For this review, take the finished solid that the model builds, in its own axes (mm). A direction names the side the tool comes from. Coordinates: 2 decimals unless noted, no trailing zeros. Loops run counter-clockwise (first coordinate to the right, second up) from the corner with the lowest first, then second, coordinate; pieces in that order, holes last. Notation, with made-up numbers: (-36.5, 67.25) -> (-24.5, 67.25) arc R17 ccw to (-24.5, 96.25) -> close; hole circle Ø5 at (8.25, -5.75). An arc over 180 degrees is marked (long way). One line per item, written item: value.
Autodesk Inventor part; units mm, degrees
ref_plane "YZ Plane" through (0, 0, 0) normal (1, 0, 0) x (0, 1, 0)
ref_plane "XZ Plane" through (0, 0, 0) normal (0, 1, 0) x (-1, 0, 0)
ref_plane "XY Plane" through (0, 0, 0) normal (0, 0, 1) x (1, 0, 0)
sketch "Sketch1" plane through (0, 0, 0) normal (0, 0, 1) x (1, 0, 0)
  line L0 (-15, 13.1624) -> (0, 13.1624) construction
  line L1 (-15, -13.1624) -> (-15, 13.1624) construction
  line L2 (0, -13.1624) -> (-15, -13.1624) construction
  line L3 (0, 13.1624) -> (0, -13.1624) construction
  circle A0 centre (20, -58.85) radius 1.2295 construction
  circle A1 centre (20, -38.35) radius 1.2295 construction
  circle A2 centre (42.1, -48.6) radius 1.2295 construction
  circle A3 centre (20, -48.6) radius 6 construction
  circle A4 centre (20, 0) radius 4 construction
  line L4 (40, 13.1624) -> (55, 13.1624) construction
  line L5 (40, -13.1624) -> (40, 13.1624) construction
  line L6 (55, -13.1624) -> (40, -13.1624) construction
  line L7 (55, 13.1624) -> (55, -13.1624) construction
  arc A5 (0, 0) -> (-15, 0) centre (-7.5, 0) ccw
  arc A6 (55, 0) -> (40, 0) centre (47.5, 0) ccw
  arc A7 (0, 0) -> (40, 0) centre (20, 0) ccw
  line L8 (53.51, -48.6) -> (3.95, -48.6) construction
  line L9 (20, -64.85) -> (43, -64.85)
  line L10 (55, 0) -> (55, -52.85)
  arc A8 (43, -64.85) -> (55, -52.85) centre (43, -52.85) ccw
  line L11 (4.8831, -54.5617) -> (-13.4793, -8.001)
  arc A9 (4.8831, -54.5617) -> (20, -64.85) centre (20, -48.6) ccw
  arc A10 (-15, 0) -> (-13.4793, -8.001) centre (6.8084, 0) ccw
  circle A11 centre (42.1, -48.6) radius 1.5
  arc A12 (19.1333, -36.7114) -> (18.1846, -38.7583) centre (42.1, -48.6) ccw
  arc A13 (21.7975, -38.0905) -> (20.9588, -39.9) centre (42.1, -48.6) ccw
  arc A14 (20.9609, -57.3051) -> (21.8001, -59.1144) centre (42.1, -48.6) ccw construction
  arc A15 (18.1869, -58.4474) -> (19.1362, -60.4941) centre (42.1, -48.6) ccw
  arc A16 (19.1362, -60.4941) -> (21.8001, -59.1144) centre (20.4681, -59.8042) ccw
  arc A17 (20.9609, -57.3051) -> (18.1869, -58.4474) centre (19.5739, -57.8763) ccw
  arc A18 (18.1846, -38.7583) -> (20.9588, -39.9) centre (19.5717, -39.3292) ccw
  arc A19 (21.7975, -38.0905) -> (19.1333, -36.7114) centre (20.4654, -37.401) ccw
  arc A20 (19.5739, -57.8763) -> (20.4681, -59.8042) centre (42.1, -48.6) ccw construction
  arc A21 (20.4654, -37.401) -> (19.5717, -39.3292) centre (42.1, -48.6) ccw construction
  arc A22 (20.9609, -57.3051) -> (21.8001, -59.1144) centre (42.1, -48.6) ccw
  arc A23 (13.7784, -47.3325) -> (13.7784, -49.8675) centre (39.8451, -48.6) ccw
  arc A24 (26.2637, -47.9396) -> (26.2637, -49.2604) centre (39.8451, -48.6) ccw
  arc A25 (13.7784, -49.8675) -> (26.2637, -49.2604) centre (20.021, -49.564) ccw
  arc A26 (26.2637, -47.9396) -> (13.7784, -47.3325) centre (20.021, -47.636) ccw
  arc A27 (20.021, -47.636) -> (20.021, -49.564) centre (42.1, -48.6) ccw construction
  circle A28 centre (-7.5, -9) radius 1.7295
  circle A29 centre (47.5, -9) radius 1.7295
  circle A30 centre (47.5, -9) radius 2
  circle A31 centre (-7.5, -9) radius 2
  circle A32 centre (-10.5, 0) radius 2.067
  circle A33 centre (44.5, 0) radius 2.067
  circle A34 centre (-10.5, 0) radius 2.5
  circle A35 centre (44.5, 0) radius 2.5
extrude "Extrusion1" add sketch "Sketch1" along normal blind 3 contours A7 A6 L10 A8 L9 A9 L11 A10 A5
properties part number "motor plate"
1. To check wall thickness, follow probe 1 along X at (y, z) = (-9.5, 2.2); probe 2 along Y at (x, z) = (18, 1.25); probe 3 along X at (y, z) = (-48, 0.75). State the ranges of each line that lie inside material, in increasing order. Write a range as from..to.
Return value:
probe 1: x = -12.89..-9.44, -5.56..2.4, 37.6..45.56, 49.44..55
probe 2: y = -64.73..-55.48, -41.72..-19.9
probe 3: x = 2.3..13.75, 26.26..40.73, 43.47..55
2. Take a section at A-A, the plane y = -5. Give the boundary of the cut face in (x, z).
Return value:
outline: (-14.42, 0) -> (0.64, 0) -> (0.64, 3) -> (-14.42, 3) -> close; (39.36, 0) -> (55, 0) -> (55, 3) -> (39.36, 3) -> close
3. Take a section at B-B, the plane x = 44.5. Give the boundary of the cut face in (y, z).
Return value:
outline: (-64.76, 0) -> (-2.5, 0) -> (-2.5, 3) -> (-64.76, 3) -> close; (2.5, 0) -> (6.87, 0) -> (6.87, 3) -> (2.5, 3) -> close
4. Take a section at C-C, the plane z = 1.45. Give the number of separate pieces and of enclosed holes in the cut face, and give its area (3 significant figures).
Return value:
separate pieces: 1
enclosed holes: 8
area: 3,060 mm2
5. For faces 4 (the cylindrical face through (21.367, -58.232, 1.479)), 5 (the flat face through (27, -28, 0)), list the 3-axis set-ups (+Z, -Z, +X, -X, +Y, -Y) from which the entire face can be reached by the end or side of a thin tool; tool diameter is ignored.
Return value:
face 4: +Z, -Z
face 5: -Z, +X, -X, +Y, -Y
6. Insertion check: pin 1 Ø1.5 at (x, y) = (6, -12) entering from -Z; pin 2 Ø5 at (x, y) = (47.5, -9) entering from +Z; pin 3 Ø1 at (y, z) = (-22, 0.5) entering from -X. Each pin has a flat end and moves straight along its axis. Give the tip position at first contact, or say it passes through.
Return value:
pin 1: passes through
pin 2: stops at z = 3
pin 3: stops at x = -8.16
7. The part is to be moulded in two halves that separate along Y. For faces 1 (the cylindrical face through (19.03, -40.73, 1.48)), 2 (the cylindrical face through (20, -20, 1)), 3 (the cylindrical face through (51.58, -61.24, 1.48)), say which applies: pulls with the +Y half, pulls with the -Y half, needs draft (parallel to the pull), parting line crosses it, or undercut.
Return value:
face 1: undercut
face 2: pulls with the +Y half
face 3: pulls with the -Y half
8. Take a section at D-D, the plane x = 31.5. Give the boundary of the cut face in (y, z), and give its area (3 significant figures).
Return value:
outline: (-64.85, 0) -> (-16.36, 0) -> (-16.36, 3) -> (-64.85, 3) -> close
area: 145 mm2
